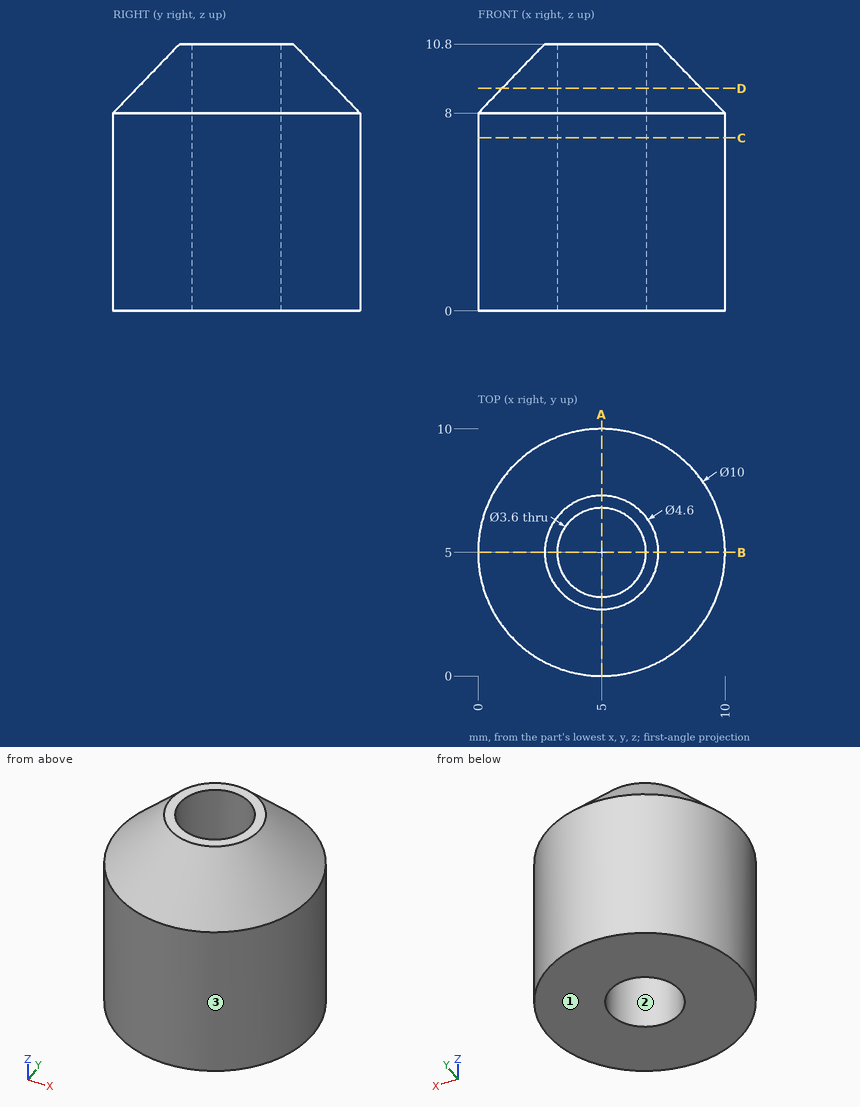
Drawing for the job (mm, zero at the part's lowest x, y, z). Round coordinates to 2 decimals unless told otherwise and drop trailing zeros. Loops run counter-clockwise (first coordinate to the right, second up) from the corner with the lowest first, then second, coordinate; pieces in that order, holes last. Notation, with made-up numbers: M 88,21.5 L 113,21.5 A18 cw 113,30.5 Z; hole C 76.5,43.25 d8. An arc over 180 degrees is marked long. Use a Markdown table: item, result. Add a question column.
(1) Cut at C-C (z = 7). Give the cut face in (x, y).
(2) Cut at A-A (x = 5). Give the cut face in (y, z), and give its area (3 significant figures).
(3) Flat gauge pins, fed straight in: pin 1 (6 mm diameter, centred on x = 8.5, y = 3, fed in from -Z); pin 2 (3 mm diameter, centred on x = 5, y = 5, fed in from -Z); pin 3 (1 mm diameter, centred on x = 6.5, z = 4.5, fed in from +Y); pin 4 (1.5 mm diameter, centred on x = 3.5, y = 8, fed in from +Z). Where does each tip first touch, or does it go through?
(4) Pull direction X, two halves, no side cores. Call the marked faces 1, 2 and 3: +X half, -X half, draft (parallel to the pull), parting line (faces both ways), or undercut.
(5) Cut at D-D (z = 9). Give the cut face in (x, y), and give its area (3 significant figures).
(6) Drill centre lines: line 1 (Y direction, x = 5, z = 3.75); line 2 (Y direction, x = 4.25, z = 4); line 3 (X direction, y = 5.5, z = 6). Where is each one in solid material? Low to high.
Geometry says:
| question | item | result |
|---|---|---|
| 1 | outline | C 5,5 d10; hole C 5,5 d3.6 |
| 2 | outline | M 0,0 L 3.2,0 L 3.2,10.8 L 2.7,10.8 L 0,8 Z; M 6.8,0 L 10,0 L 10,8 L 7.3,10.8 L 6.8,10.8 Z |
| 2 | area | 61.6 mm² |
| 3 | pin 1 | stops at z = 0 |
| 3 | pin 2 | passes through |
| 3 | pin 3 | stops at y = 9.9 |
| 3 | pin 4 | stops at z = 10.48 |
| 4 | face 1 | draft |
| 4 | face 2 | undercut |
| 4 | face 3 | parting line |
| 5 | outline | C 5,5 d8.07; hole C 5,5 d3.6 |
| 5 | area | 41.0 mm² |
| 6 | line 1 | y = 0 to 3.2, 6.8 to 10 |
| 6 | line 2 | y = 0.06 to 3.36, 6.64 to 9.94 |
| 6 | line 3 | x = 0.03 to 3.27, 6.73 to 9.97 |
